Can you work these out from the model? Positions are in its coordinate system, mm. Coordinates: 2 decimals unless noted, no trailing zeros. Write each loop counter-clockwise with the first axis right and the second up, starting at its lowest first coordinate (ties: lowest second). Pieces come first, ordered by that corner, then holes. Notation, with made-up numbers: (13, 11.5) -> (22, 11.5) arc R24 ccw to (22, 45.5) -> close; hole circle Ø11 at (50, 75.25). An arc over 180 degrees is marked (long way). Use one line per item in the form item = value.
```python
from build123d import *

# Parameters (mm, degrees)
F0_R     = 62.62304
F1_DEPTH = 43.373577
F2_R     = 53.368625
F3_DEPTH = 5.646907
F4_R     = 51.187799
F5_DEPTH = 64.743372
F6_R     = 5.08
F7_R     = 5.08
F8_R     = 5.08


with BuildPart() as f1:
    # F0 (on Top) → F1 (new body)
    with BuildSketch(Plane.XY):
        Circle(F0_R)
    extrude(amount=F1_DEPTH)

    # F2 (on face) → F3 (join)
    with BuildSketch(Plane(origin=(0, 0, 0), x_dir=(1, 0, 0), z_dir=(0, 0, -1))):
        Circle(F2_R)
    extrude(amount=-F3_DEPTH)

    # F4 (on face) → F5 (cut)
    with BuildSketch(Plane(origin=(0, 0, 0), x_dir=(1, 0, 0), z_dir=(0, 0, -1))):
        Circle(F4_R)
    extrude(amount=-F5_DEPTH, mode=Mode.SUBTRACT)

    # F6
    f6_edges = [f1.edges().sort_by_distance(p)[0] for p in [
        (-62.62304, 0, 43.373577),
    ]]
    fillet(f6_edges, radius=F6_R)

    # F7
    f7_edges = [f1.edges().sort_by_distance(p)[0] for p in [
        (-51.187799, 0, 0),
        (-51.187799, 0, 43.373577),
    ]]
    fillet(f7_edges, radius=F7_R)

    # F8
    f8_edges = [f1.edges().sort_by_distance(p)[0] for p in [
        (-62.62304, 0, 0),
    ]]
    fillet(f8_edges, radius=F8_R)


solid = f1.part
```
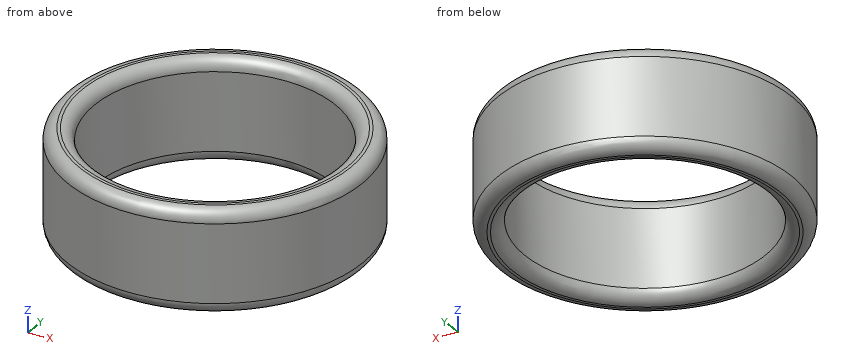
Q1. Suppose I cut it at C-C (z = 22.5). Write out the boundary of the cut face in (x, y), then the cut area to 3 significant figures.
Return value:
outline = circle Ø125.25 at (0, 0); hole circle Ø102.38 at (0, 0)
area = 4,090 mm2
Q2. If I drill on line 1 (Y direction, x = 0, z = 30); line 2 (X direction, y = -30, z = 40.5); line 3 (Y direction, x = 24, z = 35), over which ranges is the centre line in solid material (lowest first)? Write a range as from..to.
Return value:
line_1 = -62.62..-51.19, 51.19..62.62
line_2 = -54.39..-42.1, 42.1..54.39
line_3 = -57.84..-45.21, 45.21..57.84
Q3. Suppose I cut it at A-A (x = 0). Write out the boundary of the cut face in (y, z), then the cut area to 3 significant figures.
Return value:
outline = (-62.62, 5.08) arc R5.08 ccw to (-57.54, 0) -> (-56.27, 0) arc R5.08 ccw to (-51.19, 5.08) -> (-51.19, 38.29) arc R5.08 ccw to (-56.27, 43.37) -> (-57.54, 43.37) arc R5.08 ccw to (-62.62, 38.29) -> close; (51.19, 5.08) arc R5.08 ccw to (56.27, 0) -> (57.54, 0) arc R5.08 ccw to (62.62, 5.08) -> (62.62, 38.29) arc R5.08 ccw to (57.54, 43.37) -> (56.27, 43.37) arc R5.08 ccw to (51.19, 38.29) -> close
area = 948 mm2
Q4. Will these pins go through, and if not, where does the flat tip stop? pin 1 (3 mm diameter, centred on y = -11, z = 25, fed in from +X); pin 2 (5 mm diameter, centred on y = 31, z = 21.5, fed in from -X); pin 3 (2 mm diameter, centred on y = -11, z = 11.5, fed in from +X).
Return value:
pin_1 = 61.9
pin_2 = -55.76
pin_3 = 61.82
